from build123d import *

# Parameters (mm, degrees)
F0_R     = 110
F1_DEPTH = 2000
F3_DEPTH = 25
F5_DEPTH = 25


with BuildPart() as f1:
    # F0 (on Top) → F1 (new body)
    with BuildSketch(Plane.XY):
        Circle(F0_R)
    extrude(amount=F1_DEPTH)

    # F2 (on face) → F3 (join)
    with BuildSketch(Plane(origin=(0, 0, 0), x_dir=(1, 0, 0), z_dir=(0, 0, -1))):
        Polygon((130, -75.055535), (130, 75.055535), (0, 150.11107), (-130, 75.055535), (-130, -75.055535), (0, -150.11107), align=None)
    extrude(amount=-F3_DEPTH)

    # F4 (on face) → F5 (join)
    with BuildSketch(Plane.XY.offset(2000)):
        Polygon((130, -75.055535), (130, 75.055535), (0, 150.11107), (-130, 75.055535), (-130, -75.055535), (0, -150.11107), align=None)
    extrude(amount=-F5_DEPTH)


solid = f1.part
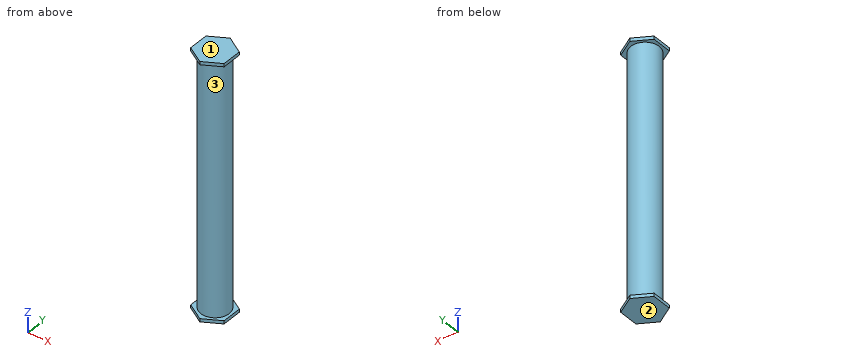
Work out the finished part from the listing and answer in its coordinate system (mm). Face numbers are marked on the shaded views. Coordinates: 2 decimals unless noted, no trailing zeros. Loops run counter-clockwise (first coordinate to the right, second up) from the corner with the lowest first, then second, coordinate; pieces in that order, holes last. Notation, with made-up numbers: (60, 27) -> (93, 27) arc R15 ccw to (93, 41) -> close; hole circle Ø9 at (52, -19). An arc over 180 degrees is marked (long way). Write each question's results on one line, items separated by ' | '. Start each with the question number.
1) Flat-ended cylindrical pins translate along their axes: P1, Ø12, axis at y = -2.5, z = 1758, coming from the +X side; P2, Ø3, axis at y = 28, z = 540, coming from the +X side; P3, Ø10, axis at y = -15, z = 1294, coming from the -X side. Find the tip coordinate at first contact, or state that the pin passes through.
2) Find section C-C on z = 584. Determine the outline of the cut face in (x, y).
3) Find section A-A on y = 0. Determine the outline of the cut face in (x, z), then the cut area to 3 significant figures.
4) The mould has two halves that part along Z. Classify the marked faces 1, 2 and 3: pulls with the +Z half, pulls with the -Z half, needs draft (parallel to the pull), parting line crosses it, or undercut.
5) Find section B-B on x = 91. Determine the outline of the cut face in (y, z).
6) Consider line 1 along Z through (x, y) = (113, 75); line 2 along X through (y, z) = (2, 1774.5); line 3 along Y through (x, z) = (8, 792). Determine where each line is inside the solid, lowest interval first.
Response values:
1) P1: stops at x = 110 | P2: stops at x = 106.76 | P3: stops at x = -109.54
2) outline: circle Ø220 at (0, 0)
3) outline: (-130, 0) -> (130, 0) -> (130, 25) -> (110, 25) -> (110, 1975) -> (130, 1975) -> (130, 2000) -> (-130, 2000) -> (-130, 1975) -> (-110, 1975) -> (-110, 25) -> (-130, 25) -> close | area: 442,000 mm^2
4) face 1: pulls with the +Z half | face 2: pulls with the -Z half | face 3: undercut
5) outline: (-97.57, 0) -> (97.57, 0) -> (97.57, 25) -> (61.8, 25) -> (61.8, 1975) -> (97.57, 1975) -> (97.57, 2000) -> (-97.57, 2000) -> (-97.57, 1975) -> (-61.8, 1975) -> (-61.8, 25) -> (-97.57, 25) -> close
6) line 1: z = 0 to 25, 1975 to 2000 | line 2: x = -109.98 to 109.98 | line 3: y = -109.71 to 109.71
